```python
from build123d import *

# Parameters (mm, degrees)
IZIM1_R                             = 62.2
Y_KSEKLIK_EKSTR_ZYON1_DEPTH         = 10
M3X0_5_HELISARMAL_IN_DI_LI_DELIK2_D = 3.15
DAIRESEL_KAPLAMA1_COUNT             = 3
IZIM5_R                             = 5
KES_EKSTR_ZYON1_DEPTH               = 10
IZIM6_R                             = 2.25
KES_EKSTR_ZYON2_DEPTH               = 10
DAIRESEL_KAPLAMA2_COUNT             = 4


with BuildPart() as part:
    # Çizim1 → Yükseklik-Ekstrüzyon1 (new body)
    with BuildSketch(Plane.XY):
        Circle(IZIM1_R)
    extrude(amount=Y_KSEKLIK_EKSTR_ZYON1_DEPTH)

    # M3x0.5 Helisarmal İçin Dişli Delik2 (through all)
    with Locations(Plane.XY.offset(10)):
        with Locations((38.32518754, 38.32518754)):
            m3x0_5_helisarmal_in_di_li_delik2 = Hole(M3X0_5_HELISARMAL_IN_DI_LI_DELIK2_D / 2)

    # Dairesel Kaplama1: M3x0.5 Helisarmal İçin Dişli Delik2 ×3 about axis
    dairesel_kaplama1_axis = Axis((0, 0, 0), (0, 0, 1))
    for i in range(1, DAIRESEL_KAPLAMA1_COUNT):
        add(m3x0_5_helisarmal_in_di_li_delik2.rotate(dairesel_kaplama1_axis, i * 360 / DAIRESEL_KAPLAMA1_COUNT), mode=Mode.SUBTRACT)

    # Çizim5 → Kes-Ekstrüzyon1 (cut)
    with BuildSketch(Plane.XY.offset(10)):
        with Locations((-37.818561572, 26.099021067)):
            Circle(IZIM5_R)
    extrude(amount=-KES_EKSTR_ZYON1_DEPTH, mode=Mode.SUBTRACT)

    # Çizim6 → Kes-Ekstrüzyon2 (cut)
    with BuildSketch(Plane.XY.offset(10)):
        with Locations((30, -25)):
            Circle(IZIM6_R)
        with Locations((-30, -25)):
            Circle(IZIM6_R)
    extrude(amount=-KES_EKSTR_ZYON2_DEPTH, mode=Mode.SUBTRACT)

    # Çizim10 → M4x0.7 Helisarmal İçin Dişli Delik4 (revolve, cut)
    with BuildSketch(Plane(origin=(0, 62.2, 5), x_dir=(0, 0, 1), z_dir=(1, 0, 0))):
        Polygon((0, 0), (0, 13.5618073), (2.1, 12.3), (2.1, 0), align=None)
    m4x0_7_helisarmal_in_di_li_delik4 = revolve(axis=Axis((0, 68.55, 5), (0, -1, 0)), mode=Mode.SUBTRACT)

    # Dairesel Kaplama2: M4x0.7 Helisarmal İçin Dişli Delik4 ×4 about axis
    dairesel_kaplama2_axis = Axis((0, 0, 0), (0, 0, 1))
    for i in range(1, DAIRESEL_KAPLAMA2_COUNT):
        add(m4x0_7_helisarmal_in_di_li_delik4.rotate(dairesel_kaplama2_axis, i * 360 / DAIRESEL_KAPLAMA2_COUNT), mode=Mode.SUBTRACT)


solid = part.part
```
Check sheet for the modelled part. Datum: model origin and axes. Units: mm. A direction names the side the tool comes from. Give positions to 0.01 mm unless a question says otherwise; leave off trailing zeros. Order: outer loops, then holes, each group sorted by start corner. A loop starts at its lowest first (then second) coordinate and runs counter-clockwise, first axis right, second up. Notation, with made-up numbers: (-26.75, 57.5) -> (-22.75, 57.5) arc R14 cw to (-22.75, 65.5) -> close; hole circle Ø10 at (77, 47.5). An arc over 180 degrees is marked (long way). Return JSON: item names as keys, results as strings.
1. Set-up check for faces 5 (the cylindrical face through (-56.14, 2.05, 4.54)), 6 (the cylindrical face through (56.14, -2.05, 4.54)), 7 (the cylindrical face through (2.05, 56.14, 4.54)), 8 (the cylindrical face through (-2.05, -56.14, 4.54)): record each of +Z, -Z, +X, -X, +Y, -Y from which the full face is reachable in a straight line by a thin tool's end or side.
From the geometry:
{"face 5": "-X", "face 6": "+X", "face 7": "+Y", "face 8": "-Y"}
2. Cross-section at A-A, the plane y = -25. Record the cut outline in (x, z), plus the area to 3 significant figures.
From the geometry:
{"outline": "(-56.95, 0) -> (-32.25, 0) -> (-32.25, 10) -> (-56.95, 10) -> close; (-27.75, 0) -> (27.75, 0) -> (27.75, 10) -> (-27.75, 10) -> close; (32.25, 0) -> (56.95, 0) -> (56.95, 10) -> (32.25, 10) -> close", "area": "1,050 mm^2"}
3. Mould release check, pull along Z, two halves, no side actions. Record for faces 1 (the conical face through (-48.857, -0.016, 4.636)), 2 (the flat face through (-1, 1, 0)), 3 (the conical face through (48.857, 0.016, 4.636)), 4 (the cylindrical face through (-35.131, 30.315, 5.07)): +Z half, -Z half, draft (parallel to the pull), parting line (faces both ways), or undercut.
From the geometry:
{"face 1": "undercut", "face 2": "-Z half", "face 3": "undercut", "face 4": "draft"}
4. Go/stop test with flat-tipped pins: P1, Ø4, axis at x = 0, z = 5, coming from the +Y side; P2, Ø4, axis at x = -23, z = 1.5, coming from the -Y side; P3, Ø1.5, axis at y = -9, z = 4, coming from the +X side. Record where each tip stops, or that it passes through.
From the geometry:
{"P1": "y = 49.84", "P2": "y = -58.55", "P3": "x = 61.65"}
5. Cross-section at C-C, the plane y = 52. Record the cut outline in (x, z).
From the geometry:
{"outline": "(-34.13, 0) -> (34.13, 0) -> (34.13, 10) -> (-34.13, 10) -> close; hole circle Ø4.2 at (0, 5)"}
6. Cross-section at B-B, the plane x = 30. Record the cut outline in (y, z).
From the geometry:
{"outline": "(-54.49, 0) -> (-27.25, 0) -> (-27.25, 10) -> (-54.49, 10) -> close; (-22.75, 0) -> (54.49, 0) -> (54.49, 10) -> (-22.75, 10) -> close"}
7. Material ranges on probe 1 along Z at (x, y) = (56.5, 0); probe 2 along Y at (x, z) = (30, 7.25); probe 3 along Y at (x, z) = (-31.5, 6), recorded low to high. Write a range as [from, to].
From the geometry:
{"probe 1": "[0, 2.9], [7.1, 10]", "probe 2": "[-54.49, -27.25], [-22.75, 54.49]", "probe 3": "[-53.63, -26.68], [-23.32, 53.63]"}
